```python
from build123d import *

# Parameters (mm, degrees)
CROQUIS1_R              = 5
CROQUIS1_R_2            = 7.5
SALIENTE_EXTRUIR1_DEPTH = 10
CROQUIS2_R              = 17.5
CROQUIS2_R_2            = 5
SALIENTE_EXTRUIR2_DEPTH = 20


with BuildPart() as part:
    # Croquis1 → Saliente-Extruir1 (new body)
    with BuildSketch(Plane.XY):
        with BuildLine():
            Line((-212, 17.5), (212, 17.5))
            ThreePointArc((212, 17.5), (229.5, 0), (212, -17.5))
            Line((212, -17.5), (-212, -17.5))
            ThreePointArc((-212, -17.5), (-229.5, 0), (-212, 17.5))
        make_face()
        with Locations((-212, 0)):
            Circle(CROQUIS1_R, mode=Mode.SUBTRACT)
        with Locations((212, 0)):
            Circle(CROQUIS1_R, mode=Mode.SUBTRACT)
        Circle(CROQUIS1_R_2, mode=Mode.SUBTRACT)
    extrude(amount=SALIENTE_EXTRUIR1_DEPTH)

    # Croquis2 → Saliente-Extruir2 (add)
    with BuildSketch(Plane.XY.offset(10)):
        with Locations((-212, 0)):
            Circle(CROQUIS2_R)
        with Locations((-212, 0)):
            Circle(CROQUIS2_R_2, mode=Mode.SUBTRACT)
    extrude(amount=SALIENTE_EXTRUIR2_DEPTH)


solid = part.part
```
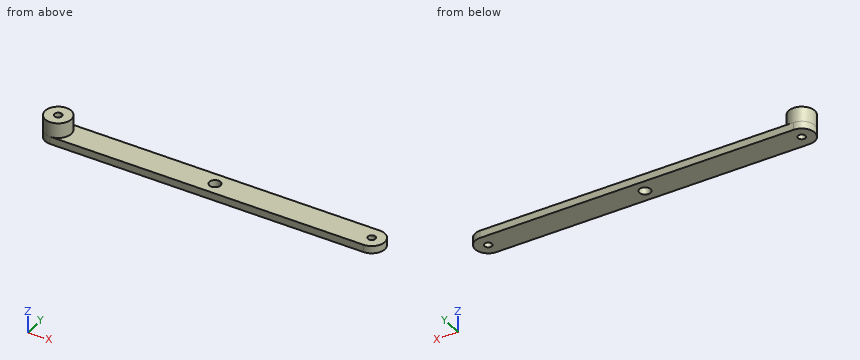
Input: part model. Units: mm. Frame: model coordinates. Give positions to 0.01 mm unless a question says otherwise; leave off trailing zeros. Order: outer loops, then holes, each group sorted by start corner. A loop starts at its lowest first (then second) coordinate and runs counter-clockwise, first axis right, second up. Notation, with made-up numbers: M 1.25,67 L 31.25,67 A34 ccw 31.25,102 Z; hole C 59,38 d3. An arc over 180 degrees is marked long. Return JSON: item names as keys, results as strings.
Item 1: Cut plane A-A (y = 0). Return loops of the section in (x, z), then the cut area to 3 significant figures.
Solutions:
{"outline": "M -229.5,0 L -217,0 L -217,30 L -229.5,30 Z; M -207,0 L -7.5,0 L -7.5,10 L -194.5,10 L -194.5,30 L -207,30 Z; M 7.5,0 L 207,0 L 207,10 L 7.5,10 Z; M 217,0 L 229.5,0 L 229.5,10 L 217,10 Z", "area": "4,740 mm^2"}
Item 2: Cut plane B-B (x = 0). Return loops of the section in (y, z).
Solutions:
{"outline": "M -17.5,0 L -7.5,0 L -7.5,10 L -17.5,10 Z; M 7.5,0 L 17.5,0 L 17.5,10 L 7.5,10 Z"}
Item 3: Cut plane D-D (x = 124). Return loops of the section in (y, z), then the cut area to 3 significant figures.
Solutions:
{"outline": "M -17.5,0 L 17.5,0 L 17.5,10 L -17.5,10 Z", "area": "350 mm^2"}
Item 4: First-contact query: P1, Ø12, axis at x = -17.5, z = 19, coming from the -Y side; P2, Ø10.5, axis at x = 113.5, y = 4, coming from the +Z side; P3, Ø6, axis at y = 13.5, z = 14, coming from the -X side; P4, Ø3, axis at y = -3.5, z = 20.5, coming from the -X side. Flat tips, straight axial feed; report the tip coordinate or a pass-through.
Solutions:
{"P1": "through", "P2": "z = 10", "P3": "x = -226", "P4": "x = -229.39"}
Item 5: Ray query, probe 1 along Y at (x, z) = (0, 7.75); probe 2 along X at (y, z) = (0.5, 20.75); probe 3 along X at (y, z) = (-2.5, 6). Return the intervals inside material, ascending.
Solutions:
{"probe 1": "-17.5 to -7.5, 7.5 to 17.5", "probe 2": "-229.49 to -216.97, -207.03 to -194.51", "probe 3": "-229.32 to -216.33, -207.67 to -7.07, 7.07 to 207.67, 216.33 to 229.32"}
Item 6: Cut plane C-C (z = 23.5). Return loops of the section in (x, y), then the cut area to 3 significant figures.
Solutions:
{"outline": "C -212,0 d35; hole C -212,0 d10", "area": "884 mm^2"}
